Autodesk Inventor part; units mm, degrees
ref_plane "YZ Plane" through (0, 0, 0) normal (1, 0, 0) x (0, 1, 0)
ref_plane "XZ Plane" through (0, 0, 0) normal (0, 1, 0) x (-1, 0, 0)
ref_plane "XY Plane" through (0, 0, 0) normal (0, 0, 1) x (1, 0, 0)
sketch "Sketch1" plane through (0, 0, 0) normal (0, 0, 1) x (1, 0, 0)
  line L0 (-259, 0) -> (259, 0) construction
  line L1 (0, -140) -> (0, 140) construction
  line L2 (-185, 100) -> (185, 100)
  line L3 (185, 100) -> (185, -100)
  line L4 (185, -100) -> (-185, -100)
  line L5 (-185, -100) -> (-185, 100)
  line L6 (175, 90) -> (-175, 90)
  line L7 (-175, 90) -> (-175, -90)
  line L8 (-175, -90) -> (175, -90)
  line L9 (175, -90) -> (175, 90)
  line L10 (-180, 95) -> (180, 95) construction
  line L11 (180, 95) -> (180, -95) construction
  line L12 (180, -95) -> (-180, -95) construction
  line L13 (-180, -95) -> (-180, 95) construction
  point P0 (0, 0)
  point P1 (0, 95)
  point P2 (180, 0)
  point P3 (0, -95)
  point P4 (-180, 0)
  point P5 (-90, 95)
  point P6 (90, 95)
  point P7 (-90, -95)
  point P8 (90, -95)
  dimension "d0" = 370
  dimension "d1" = 200
  dimension "d2" = 10
  dimension "d3" = 5
  dimension "d19" = 90
  dimension "d20" = 90
extrude "Extrusion1" add sketch "Sketch1" against normal blind 6 contours L2 L3 L4 L5 | L9 L8 L7 L6
extrude "Extrusion2" cut sketch "Sketch1" against normal blind 10 contours L9 L8 L7 L6
fillet "Fillet1" radius 5 8 edges at (-175, 90, -3) (-185, 100, -3) (185, 100, -3) (175, 90, -3) (185, -100, -3) (-185, -100, -3) (-175, -90, -3) (175, -90, -3)
chamfer "Chamfer1" distance 0.5 angle 45 16 edges at (0, 100, 0) (-183.5355, 98.5355, 0) (-185, 0, 0) (-183.5355, -98.5355, 0) (0, -100, 0) (183.5355, -98.5355, 0) (185, 0, 0) (183.5355, 98.5355, 0) (0, 90, 0) (173.5355, 88.5355, 0) (175, 0, 0) (173.5355, -88.5355, 0) (0, -90, 0) (-173.5355, -88.5355, 0) (-175, 0, 0) (-173.5355, 88.5355, 0)
hole "Hole1" at (-180, 95, 0) at (0, 95, 0) at (180, 95, 0) at (180, 0, 0) at (180, -95, 0) at (0, -95, 0) at (-180, 0, 0) at (-180, -95, 0) at (-90, 95, 0) at (90, 95, 0) at (90, -95, 0) at (-90, -95, 0) direction (0, 0, -1) diameter 4.5 end through all countersink diameter 10 countersink angle 90
properties part number "GRJ-04-106" material "Fenolite OR"
Part model, mm, in its own coordinate system. Round coordinates to 2 decimals unless told otherwise and drop trailing zeros. Loops run counter-clockwise (first coordinate to the right, second up) from the corner with the lowest first, then second, coordinate; pieces in that order, holes last. Notation, with made-up numbers: (70, 54) -> (78, 54) arc R19 ccw to (78, 80) -> close; hole circle Ø8 at (64, -15). An arc over 180 degrees is marked (long way). Use CSV: the item, a comma, the result in double quotes. Start each with the question number.
1) Cut at A-A, the plane x = 141. Write the cut outline in (y, z).
2) Cut at C-C, the plane y = 38.5. Write the cut outline in (x, z).
3) Drop flat-ended pins along their axis: P1, Ø6, axis at x = -180, y = -95, coming from the +Z side; P2, Ø7, axis at x = 90, y = -95, coming from the +Z side. Give the stop position or say it passes through.
4) Cut at B-B, the plane z = -5.05. Give the number of separate pieces and of enclosed holes in the cut face, plus the area to 3 significant figures.
5) Pull direction X, two halves, no side cores. Call faces 1 (the flat face through (44, 95, 0)), 2 (the conical face through (87.64, -94.47, -2.58)): +X half, -X half, draft (parallel to the pull), parting line (faces both ways), or undercut.
6) Wall check: L1, parallel to X at y = 0, z = -3.5; L2, parallel to Y at x = -90, z = -3.75; L3, parallel to X at y = -95, z = -4.6. Give the ranges that are in metal, low to high. Write a range as [from, to].
Determined:
1,outline,"(-100, -6) -> (-90, -6) -> (-90, -0.5) -> (-90.5, 0) -> (-99.5, 0) -> (-100, -0.5) -> close; (90, -6) -> (100, -6) -> (100, -0.5) -> (99.5, 0) -> (90.5, 0) -> (90, -0.5) -> close"
2,outline,"(-185, -6) -> (-175, -6) -> (-175, -0.5) -> (-175.5, 0) -> (-184.5, 0) -> (-185, -0.5) -> close; (175, -6) -> (185, -6) -> (185, -0.5) -> (184.5, 0) -> (175.5, 0) -> (175, -0.5) -> close"
3,P1,"stops at z = -2"
3,P2,"stops at z = -1.5"
4,separate pieces,"1"
4,enclosed holes,"13"
4,area,"10,800 mm2"
5,face 1,"draft"
5,face 2,"undercut"
6,L1,"x = [-185, -182.25], [-177.75, -175], [175, 177.75], [182.25, 185]"
6,L2,"y = [-100, -97.25], [-92.75, -90], [90, 92.75], [97.25, 100]"
6,L3,"x = [-185, -182.25], [-177.75, -92.25], [-87.75, -2.25], [2.25, 87.75], [92.25, 177.75], [182.25, 185]"
